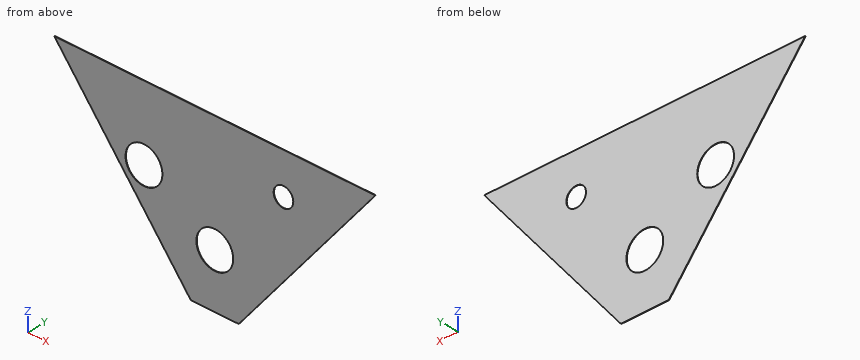
Autodesk Inventor part; units mm, degrees
ref_plane "YZ Plane" through (0, 0, 0) normal (1, 0, 0) x (0, 1, 0)
ref_plane "XZ Plane" through (0, 0, 0) normal (0, 1, 0) x (-1, 0, 0)
ref_plane "XY Plane" through (0, 0, 0) normal (0, 0, 1) x (1, 0, 0)
sketch "Sketch1" plane through (0, 0, 0) normal (0, 1, 0) x (-1, 0, 0)
  line L0 (0, 790) -> (0, 0)
  line L1 (735.0906, 788) -> (735.0906, 790)
  line L2 (735.0906, 790) -> (0, 790)
  line L3 (735.0906, 788) -> (110, 0)
  line L4 (110, 0) -> (0, 0)
  line L5 (735.9762, 809.1108) -> (102.084, 10.0153)
  point P0 (648.1236, 678.3679)
  point P1 (0, 678)
  dimension "d1" = 735.0906
  dimension "d2" = 2
  dimension "d5" = 128.424
  dimension "d6" = 110
  dimension "d9" = 790
  dimension "d28" = 128.424
extrude "Plate1" add sketch "Sketch1" along normal blind 2
mirror "Mirror1" about plane through (0, 0, 0) normal (1, 0, 0)
sketch "Sketch2" plane through (0, 0, 0) normal (0, -1, 0) x (1, 0, 0)
  line L0 (-110, 0) -> (110, 0) construction
  line L1 (-110, 0) -> (-735.0906, 788) construction
  circle A0 centre (-325, 450) radius 84.5
  line L2 (110, 0) -> (735.0906, 788) construction
  circle A1 centre (0, 250) radius 84.5
  circle A2 centre (315, 600) radius 45
  line L3 (-110, 0) -> (110, 0) construction
  line L4 (-240.5, 450) -> (-240.5, 164.5105) construction
  line L5 (-84.5, 250) -> (-84.5, 0) construction
  line L6 (84.5, 250) -> (84.5, 0) construction
  line L7 (270, 600) -> (270, 0) construction
  line L8 (-325, 534.5) -> (270, 534.5) construction
  line L9 (-325, 365.5) -> (270, 365.5) construction
  line L10 (0, 334.5) -> (270, 334.5) construction
  line L11 (315, 555) -> (270, 555) construction
  line L12 (-735.0906, 790) -> (735.0906, 790)
  line L13 (-735.0906, 788) -> (-735.0906, 790)
  line L14 (735.0906, 788) -> (735.0906, 790)
  point P0 (0, 0)
  point P1 (0, 0)
  point P2 (0, 0)
  point P3 (0, 0)
  point P4 (-84.5, 144.3746)
  point P5 (0, 0)
  point P6 (0, 0)
  dimension "d13" = 169
  dimension "d16" = 250
  dimension "d17" = 450
  dimension "d18" = 325
  dimension "d19" = 31
  dimension "d20" = 90
  dimension "d21" = 156
  dimension "d23" = 315
  dimension "d24" = 600
extrude "Extrusion1" cut sketch "Sketch2" against normal through all
sketch "Sketch3" plane through (0, 0, 0) normal (0, -1, 0) x (1, 0, 0)
  line L0 (-55, 616) -> (-55, 628) construction
  line L1 (-55, 628) -> (55, 628) construction
  line L2 (55, 628) -> (55, 616) construction
  line L3 (55, 616) -> (-55, 616) construction
  line L4 (-663.2335, 678) -> (663.2335, 678)
  point P0 (0, 0)
  point P1 (0, 616)
  point P2 (0, 678)
  dimension "d25" = 12
  dimension "d26" = 110
  dimension "d27" = 50
mark "Mark1"
equation "\"d3\" = Thickness"
equation "\"BendReliefWidth\" = Thickness"
equation "\"BendReliefDepth\" = 0.5 * Thickness"
equation "\"CornerReliefSize\" = 4 * Thickness"
equation "\"MinimumRemnant\" = 2 * Thickness"
equation "\"GapSize\" = Thickness"
properties part number "MSC 701 face 1" material "Stainless Steel"
Part model, mm, in its own coordinate system. Round coordinates to 2 decimals unless told otherwise and drop trailing zeros. Loops run counter-clockwise (first coordinate to the right, second up) from the corner with the lowest first, then second, coordinate; pieces in that order, holes last.
1. Flat gauge pin, fed straight in: pin 1 (1 mm diameter, centred on x = 345.5, y = 1.5, fed in from -Z). Where does the tip first touch, or does it go through?
Solutions:
pin 1: stops at z = 296.25
2. Drill centre lines: line 1 along Z through (x, y) = (0, 1.35); line 2 along X through (y, z) = (0.85, 623.5); line 3 along X through (y, z) = (0.5, 571). Where is each one in solid material? Low to high.
Solutions:
line 1: z = 0 to 165.5, 334.5 to 790
line 2: x = -604.6 to 276.62, 353.38 to 604.6
line 3: x = -562.95 to 280.59, 349.41 to 562.95
3. Slice it at B-B (y = 1.1). Give the cut face in (x, z), and give its area (3 significant figures).
Solutions:
outline: (-735.09, 788) - (-110, 0) - (110, 0) - (735.09, 788) - (735.09, 790) - (-735.09, 790) - close; hole circle Ø169 at (-325, 450); hole circle Ø169 at (0, 250); hole circle Ø90 at (315, 600)
area: 618,000 mm2
4. Slice it at A-A (x = 0). Give the cut face in (y, z).
Solutions:
outline: (0, 0) - (2, 0) - (2, 165.5) - (0, 165.5) - close; (0, 334.5) - (2, 334.5) - (2, 790) - (0, 790) - close
5. Slice it at C-C (z = 600). Give the cut face in (x, y), and give its area (3 significant figures).
Solutions:
outline: (-585.96, 0) - (270, 0) - (270, 2) - (-585.96, 2) - close; (360, 0) - (585.96, 0) - (585.96, 2) - (360, 2) - close
area: 2,160 mm2
6. Slice it at D-D (x = -622). Give the cut face in (y, z).
Solutions:
outline: (0, 645.44) - (2, 645.44) - (2, 790) - (0, 790) - close
